Source: three-view drawing plus pictorial views. Frame: mm from the lowest corner of the part. A direction names the side the tool comes from. Give positions to 0.01 mm unless a question says otherwise; leave off trailing zeros. Loops run counter-clockwise (first coordinate to the right, second up) from the corner with the lowest first, then second, coordinate; pieces in that order, holes last. Notation, with made-up numbers: (53.25, 8) - (92.25, 8) arc R22 ccw to (92.25, 42) - close; hole circle Ø7 at (-9, 30.25). An arc over 180 degrees is marked (long way). Put each result on its own line as item: value.
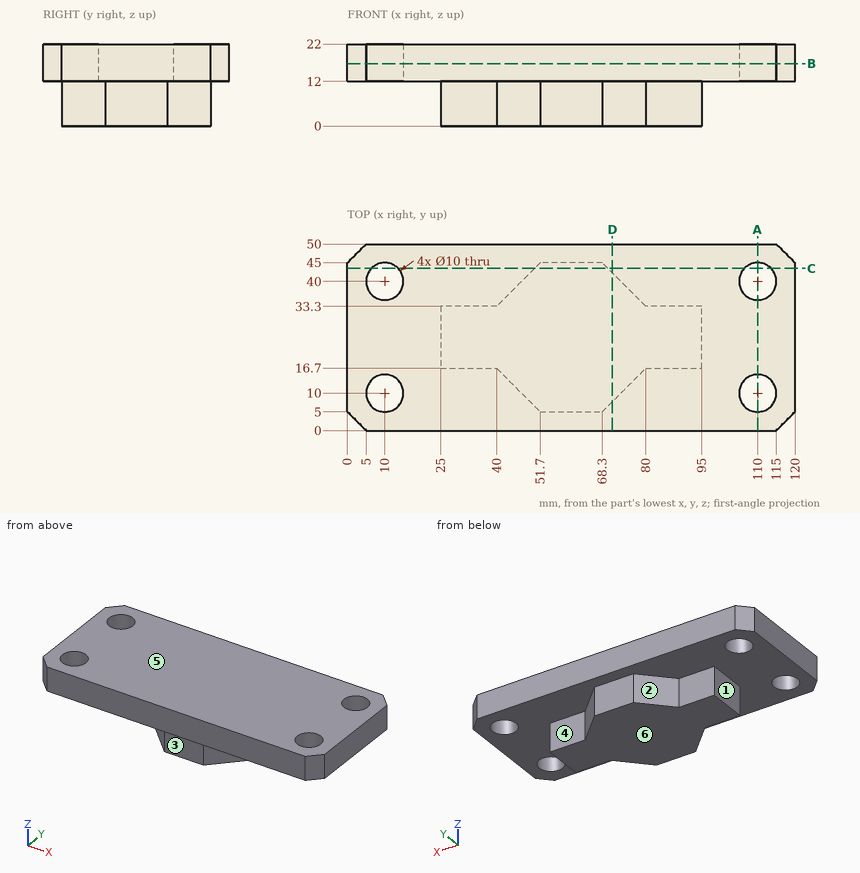
1) Material intervals for line 1 along Y through (x, z) = (10.5, 12.75); line 2 along X through (y, z) = (14.5, 14.75); line 3 along Y through (x, z) = (111.5, 14.75), sorted ascending. Write a range as [from, to].
Check result:
line 1: [0, 5.03], [14.97, 35.03], [44.97, 50]
line 2: [0, 7.82], [12.18, 107.82], [112.18, 120]
line 3: [0, 5.23], [14.77, 35.23], [44.77, 50]
2) Section query C-C, the plane y = 43.5. Output: boundary loops of the cut face in (x, z), plus the area to 3 significant figures.
Check result:
outline: (0, 12) - (6.43, 12) - (6.43, 22) - (0, 22) - close; (13.57, 12) - (50.2, 12) - (50.2, 0) - (69.8, 0) - (69.8, 12) - (106.43, 12) - (106.43, 22) - (13.57, 22) - close; (113.57, 12) - (120, 12) - (120, 22) - (113.57, 22) - close
area: 1,290 mm²
3) Section query A-A, the plane x = 110. Output: boundary loops of the cut face in (y, z), plus the area to 3 significant figures.
Check result:
outline: (0, 12) - (5, 12) - (5, 22) - (0, 22) - close; (15, 12) - (35, 12) - (35, 22) - (15, 22) - close; (45, 12) - (50, 12) - (50, 22) - (45, 22) - close
area: 300 mm²
4) Mould query, pull axis Z, two halves, no side actions, for the marked faces 4, 5 and 6. Classes: pulls with the +Z half, pulls with the -Z half, needs draft (parallel to the pull), parting line crosses it, or undercut.
Check result:
face 4: needs draft
face 5: pulls with the +Z half
face 6: pulls with the -Z half
5) Section query B-B, the plane z = 16.75. Output: boundary loops of the cut face in (x, y), plus the area to 3 significant figures.
Check result:
outline: (0, 5) - (5, 0) - (115, 0) - (120, 5) - (120, 45) - (115, 50) - (5, 50) - (0, 45) - close; hole circle Ø10 at (10, 10); hole circle Ø10 at (10, 40); hole circle Ø10 at (110, 10); hole circle Ø10 at (110, 40)
area: 5,640 mm²
6) Pin query (flat end, axial travel): P1, Ø3, axis at x = 49.5, z = 6, coming from the -Y side; P2, Ø6, axis at x = 90, z = 5, coming from the -Y side; P3, Ø6, axis at x = 10, y = 40, coming from the -Z side; P4, Ø9.5, axis at x = 60, z = 5.5, coming from the +Y side. Return the tip coordinate at first contact, or that it passes through.
Check result:
P1: y = 5.7
P2: y = 16.7
P3: through
P4: y = 45
7) Access query for the marked faces 1, 2 and 3. Directions: +Z, -Z, +X, -X, +Y, -Y. A direction counts if a zero-diameter tool reaches every point of the face in a straight line with its end or side. Return the directions, or none.
Check result:
face 1: -Z, -X, +Y, -Y
face 2: -Z, -X, +Y
face 3: -Z, +X, -X, -Y
8) Section query D-D, the plane x = 71. Output: boundary loops of the cut face in (y, z).
Check result:
outline: (0, 12) - (7.7, 12) - (7.7, 0) - (42.3, 0) - (42.3, 12) - (50, 12) - (50, 22) - (0, 22) - close
